Read the model definition and answer for the solid it produces. Units are mm, in the model's axes. A direction names the side the tool comes from. Give positions to 0.01 mm unless a question says otherwise; leave off trailing zeros. Write each loop counter-clockwise with the first axis right and the second up, starting at its lowest first coordinate (ties: lowest second). Pieces come first, ordered by that corner, then holes.
```python
from build123d import *

# Parameters (mm, degrees)
EXTRUDE_1_DEPTH     = 68
SKETCH_2_W          = 49.215089209
SKETCH_2_H          = 60
CUT_EXTRUDE_1_DEPTH = 60
SKETCH_3_R          = 7.815290935
CUT_EXTRUDE_2_DEPTH = 68
SKETCH_3_4_R        = 7.815290935
CUT_EXTRUDE_3_DEPTH = 68
SKETCH_5_W          = 5.029333187
SKETCH_5_H          = 40
EXTRUDE_2_DEPTH     = 61


with BuildPart() as part:
    # Эскиз1 → Бобышка-Вытянуть1 (new body)
    with BuildSketch(Plane.XY):
        with BuildLine():
            Line((-90, 60), (-10, 60))
            ThreePointArc((-10, 60), (-2.928932188, 57.071067812), (0, 50))
            Line((0, 50), (0, 10))
            ThreePointArc((0, 10), (-2.928932188, 2.928932188), (-10, 0))
            Line((-10, 0), (-90, 0))
            ThreePointArc((-90, 0), (-97.071067812, 2.928932188), (-100, 10))
            Line((-100, 10), (-100, 50))
            ThreePointArc((-100, 50), (-97.071067812, 57.071067812), (-90, 60))
        make_face()
    extrude(amount=EXTRUDE_1_DEPTH)

    # Эскиз2 → Вырез-Вытянуть1 (cut)
    with BuildSketch(Plane(origin=(0, 60, 0), x_dir=(1, 0, 0), z_dir=(0, 1, 0))):
        with Locations((-12.715841509, -34)):
            Rectangle(SKETCH_2_W, SKETCH_2_H)
        with Locations((-87.284158491, -34)):
            Rectangle(SKETCH_2_W, SKETCH_2_H)
    extrude(amount=-CUT_EXTRUDE_1_DEPTH, mode=Mode.SUBTRACT)

    # Эскиз3 → Вырез-Вытянуть2 (cut)
    with BuildSketch(Plane(origin=(0, 0, 0), x_dir=(-1, 0, 0), z_dir=(0, 0, -1))):
        with Locations((22.08824666, 30)):
            Circle(SKETCH_3_R)
    extrude(amount=-CUT_EXTRUDE_2_DEPTH, mode=Mode.SUBTRACT)

    # Эскиз3<4> → Вырез-Вытянуть3 (cut)
    with BuildSketch(Plane(origin=(0, 0, 0), x_dir=(-1, 0, 0), z_dir=(0, 0, -1))):
        with Locations((77.91175334, 30)):
            Circle(SKETCH_3_4_R)
        with Locations((22.08824666, 30)):
            Circle(SKETCH_3_4_R)
    extrude(amount=-CUT_EXTRUDE_3_DEPTH, mode=Mode.SUBTRACT)

    # Эскиз5 → Бобышка-Вытянуть2 (add)
    with BuildSketch(Plane(origin=(0, 0, 0), x_dir=(-1, 0, 0), z_dir=(0, 0, -1))):
        with Locations((2.514666594, 30)):
            Rectangle(SKETCH_5_W, SKETCH_5_H)
        with Locations((97.485333407, 30)):
            Rectangle(SKETCH_5_W, SKETCH_5_H)
    extrude(amount=EXTRUDE_2_DEPTH)


solid = part.part
```
Item 1: Each of these flat-tipped pins is pushed along its axis until it touches: pin 1 Ø12.5 at (x, y) = (-77.91, 30) entering from +Z; pin 2 Ø25 at (x, y) = (-22.09, 30) entering from -Z; pin 3 Ø2.5 at (x, z) = (-1.5, -21) entering from +Y; pin 4 Ø1 at (y, z) = (14, 34.5) entering from +X. Where does it stop, or does it pass through?
Result set:
pin 1: passes through
pin 2: stops at z = 0
pin 3: stops at y = 50
pin 4: stops at x = -37.32
Item 2: Which of the six approach directions +Z, -Z, +X, -X, +Y, -Y give full straight-line access (tool end or side, diameter ignored) to faces 5 (the flat face through (-15, 24, 4)), 6 (the flat face through (-86, 30, 64)), 7 (the flat face through (-5.029, 30, -30))?
Result set:
face 5: +X, +Y, -Y
face 6: -X, +Y, -Y
face 7: -Z, +Y, -Y
Item 3: Find the intervals of material crossed by line 1 along Z through (x, y) = (-68, 9.5); line 2 along Z through (x, y) = (-42, 14.5); line 3 along X through (y, z) = (18, -2.5), in increasing order.
Result set:
line 1: z = 0 to 4, 64 to 68
line 2: z = 0 to 68
line 3: x = -100 to -94.97, -5.03 to 0
Item 4: Section B-B (y = 30) is taken. Give the number of separate pieces and of enclosed holes in the cut face, and give its area (3 significant figures).
Result set:
separate pieces: 5
enclosed holes: 0
area: 2,680 mm2
Item 5: Section A-A (z = -20) is taken. Write down the section's boundary in (x, y).
Result set:
outline: (-100, 10) - (-94.97, 10) - (-94.97, 50) - (-100, 50) - close; (-5.03, 10) - (0, 10) - (0, 50) - (-5.03, 50) - close
Item 6: Section D-D (y = 5.5) is taken. Write down the section's boundary in (x, z), and give its area (3 significant figures).
Result set:
outline: (-98.93, 0) - (-1.07, 0) - (-1.07, 4) - (-37.32, 4) - (-37.32, 64) - (-1.07, 64) - (-1.07, 68) - (-98.93, 68) - (-98.93, 64) - (-62.68, 64) - (-62.68, 4) - (-98.93, 4) - close
area: 2,300 mm2
Item 7: Determine the mould class of faces 1 (the cylindrical face through (-96.99, 2.85, 65.97)), 2 (the cylindrical face through (-85.366, 32.348, 1.972)), 3 (the flat face through (-49, 30, 68)), 4 (the cylindrical face through (-3.01, 57.15, 65.97)) for opening direction X: pulls with the +X half, pulls with the -X half, needs draft (parallel to the pull), parting line crosses it, or undercut.
Result set:
face 1: pulls with the -X half
face 2: undercut
face 3: needs draft
face 4: pulls with the +X half
Item 8: Section C-C (x = -77) is taken. Write down the section's boundary in (y, z), and give its area (3 significant figures).
Result set:
outline: (0, 0) - (22.24, 0) - (22.24, 4) - (0, 4) - close; (0, 64) - (22.24, 64) - (22.24, 68) - (0, 68) - close; (37.76, 0) - (60, 0) - (60, 4) - (37.76, 4) - close; (37.76, 64) - (60, 64) - (60, 68) - (37.76, 68) - close
area: 356 mm2
